Can you work these out from the model? Positions are in its coordinate system, mm. Face numbers are marked on the shaded views. A direction names the side the tool comes from. Coordinates: 2 decimals unless noted, no trailing zeros. Order: outer loops, then holes, each group sorted by start corner. A loop starts at its lowest first (then second) coordinate and runs counter-clockwise, first axis right, second up. Notation, with made-up numbers: (-0.5, 77) -> (34.5, 77) arc R17 cw to (34.5, 87) -> close; hole circle Ø6 at (-22.75, -5). An arc over 180 degrees is marked (long way). Write item = value, one per line.
```python
from build123d import *

# Parameters (mm, degrees)
SKETCH1_W                        = 100
SKETCH1_H                        = 130
BASE_FLANGE1_DEPTH               = 0.7366
BOX_REAR_STRIP_W                 = 4.4196
BOX_REAR_STRIP_H                 = 0.7366
BOX_REAR_STRIP_CUT_DEPTH         = 100
BOX_REAR_DEPTH                   = 100
BOX_FRONT_STRIP_W                = 4.4196
BOX_FRONT_STRIP_H                = 0.7366
BOX_FRONT_STRIP_CUT_DEPTH        = 100
BOX_FRONT_DEPTH                  = 100
BOX_FRONT_TABS_STRIP_W           = 4.4196
BOX_FRONT_TABS_STRIP_H           = 0.7366
BOX_FRONT_TABS_STRIP_CUT_DEPTH   = 59.2634
BOX_FRONT_TABS_STRIP_2_W         = 4.4196
BOX_FRONT_TABS_STRIP_2_H         = 0.7366
BOX_FRONT_TABS_STRIP_CUT_2_DEPTH = 59.2634
BOX_FRONT_TABS_DEPTH             = 59.2634
BOX_FRONT_TABS_BEND_DEPTH        = 59.2634
BOX_REAR_TABS_STRIP_W            = 4.4196
BOX_REAR_TABS_STRIP_H            = 0.7366
BOX_REAR_TABS_STRIP_CUT_DEPTH    = 59.2634
BOX_REAR_TABS_STRIP_2_W          = 4.4196
BOX_REAR_TABS_STRIP_2_H          = 0.7366
BOX_REAR_TABS_STRIP_CUT_2_DEPTH  = 59.2634
BOX_REAR_TABS_DEPTH              = 59.2634
BOX_REAR_TABS_BEND_DEPTH         = 59.2634
EDGE_FLANGE6_DEPTH               = 128.5268
EDGE_FLANGE6_START               = 0.7366
EDGE_FLANGE6_FLAT_DEPTH          = 0.7366
EDGE_FLANGE6_BEND_DEPTH          = 128.5268
EDGE_FLANGE6_FLAT_2_DEPTH        = 0.7366


# Sheet-metal steps are written as plain solids
with BuildPart() as part:
    # Sketch1 → Base-Flange1 (new body)
    with BuildSketch(Plane(origin=(0, 0, 0), x_dir=(1, 0, 0), z_dir=(0, 1, 0))):
        Rectangle(SKETCH1_W, SKETCH1_H)
    extrude(amount=-BASE_FLANGE1_DEPTH)

    # Box rear strip (across the edge) → Box rear strip cut (cut)
    with BuildSketch(Plane(origin=(50, 0, -65), x_dir=(0, 0, 1), z_dir=(-1, 0, 0))):
        with Locations((-1.4732, -0.3683)):
            Rectangle(BOX_REAR_STRIP_W, BOX_REAR_STRIP_H)
    extrude(amount=BOX_REAR_STRIP_CUT_DEPTH, mode=Mode.SUBTRACT)

    # Box rear section (across the edge) → Box rear (add)
    with BuildSketch(Plane(origin=(50, 0, -65), x_dir=(0, 0, 1), z_dir=(-1, 0, 0))):
        with BuildLine():
            Line((-0.7366, 0.7366), (-0.7366, 60))
            Line((-0.7366, 60), (0, 60))
            Line((0, 60), (0, 0.7366))
            ThreePointArc((0, 0.7366), (0.215745145, 0.215745145), (0.7366, 0))
            Line((0.7366, 0), (0.7366, -0.7366))
            ThreePointArc((0.7366, -0.7366), (-0.30510971, -0.30510971), (-0.7366, 0.7366))
        make_face()
    extrude(amount=BOX_REAR_DEPTH)

    # Box front strip (across the edge) → Box front strip cut (cut)
    with BuildSketch(Plane(origin=(-50, 0, 65), x_dir=(0, 0, -1), z_dir=(1, 0, 0))):
        with Locations((-1.4732, -0.3683)):
            Rectangle(BOX_FRONT_STRIP_W, BOX_FRONT_STRIP_H)
    extrude(amount=BOX_FRONT_STRIP_CUT_DEPTH, mode=Mode.SUBTRACT)

    # Box front section (across the edge) → Box front (add)
    with BuildSketch(Plane(origin=(-50, 0, 65), x_dir=(0, 0, -1), z_dir=(1, 0, 0))):
        with BuildLine():
            Line((-0.7366, 0.7366), (-0.7366, 60))
            Line((-0.7366, 60), (0, 60))
            Line((0, 60), (0, 0.7366))
            ThreePointArc((0, 0.7366), (0.215745145, 0.215745145), (0.7366, 0))
            Line((0.7366, 0), (0.7366, -0.7366))
            ThreePointArc((0.7366, -0.7366), (-0.30510971, -0.30510971), (-0.7366, 0.7366))
        make_face()
    extrude(amount=BOX_FRONT_DEPTH)

    # Box-front tabs strip (across the edge) → Box-front tabs strip cut (cut)
    with BuildSketch(Plane(origin=(-50, 0.7366, 65), x_dir=(1, 0, 0), z_dir=(0, 1, 0))):
        with Locations((-1.4732, -0.3683)):
            Rectangle(BOX_FRONT_TABS_STRIP_W, BOX_FRONT_TABS_STRIP_H)
    extrude(amount=BOX_FRONT_TABS_STRIP_CUT_DEPTH, mode=Mode.SUBTRACT)

    # Box-front tabs strip 2 (across the edge) → Box-front tabs strip cut 2 (cut)
    with BuildSketch(Plane(origin=(50, 60, 65), x_dir=(-1, 0, 0), z_dir=(0, -1, 0))):
        with Locations((-1.4732, -0.3683)):
            Rectangle(BOX_FRONT_TABS_STRIP_2_W, BOX_FRONT_TABS_STRIP_2_H)
    extrude(amount=BOX_FRONT_TABS_STRIP_CUT_2_DEPTH, mode=Mode.SUBTRACT)

    # Box-front tabs section (across the edge) → Box-front tabs (add)
    with BuildSketch(Plane(origin=(-50, 0.7366, 65), x_dir=(1, 0, 0), z_dir=(0, 1, 0))):
        with BuildLine():
            Line((-0.7366, 0.7366), (-0.7366, 10))
            Line((-0.7366, 10), (0, 10))
            Line((0, 10), (0, 0.7366))
            ThreePointArc((0, 0.7366), (0.215745145, 0.215745145), (0.7366, 0))
            Line((0.7366, 0), (0.7366, -0.7366))
            ThreePointArc((0.7366, -0.7366), (-0.30510971, -0.30510971), (-0.7366, 0.7366))
        make_face()
    extrude(amount=BOX_FRONT_TABS_DEPTH)

    # Box-front tabs section 2 (across the edge) → Box-front tabs bend (add)
    with BuildSketch(Plane(origin=(50, 60, 65), x_dir=(-1, 0, 0), z_dir=(0, -1, 0))):
        with BuildLine():
            Line((-0.7366, 0.7366), (-0.7366, 10))
            Line((-0.7366, 10), (0, 10))
            Line((0, 10), (0, 0.7366))
            ThreePointArc((0, 0.7366), (0.215745145, 0.215745145), (0.7366, 0))
            Line((0.7366, 0), (0.7366, -0.7366))
            ThreePointArc((0.7366, -0.7366), (-0.30510971, -0.30510971), (-0.7366, 0.7366))
        make_face()
    extrude(amount=BOX_FRONT_TABS_BEND_DEPTH)

    # Box-rear tabs strip (across the edge) → Box-rear tabs strip cut (cut)
    with BuildSketch(Plane(origin=(50, 0.7366, -65), x_dir=(-1, 0, 0), z_dir=(0, 1, 0))):
        with Locations((-1.4732, -0.3683)):
            Rectangle(BOX_REAR_TABS_STRIP_W, BOX_REAR_TABS_STRIP_H)
    extrude(amount=BOX_REAR_TABS_STRIP_CUT_DEPTH, mode=Mode.SUBTRACT)

    # Box-rear tabs strip 2 (across the edge) → Box-rear tabs strip cut 2 (cut)
    with BuildSketch(Plane(origin=(-50, 60, -65), x_dir=(1, 0, 0), z_dir=(0, -1, 0))):
        with Locations((-1.4732, -0.3683)):
            Rectangle(BOX_REAR_TABS_STRIP_2_W, BOX_REAR_TABS_STRIP_2_H)
    extrude(amount=BOX_REAR_TABS_STRIP_CUT_2_DEPTH, mode=Mode.SUBTRACT)

    # Box-rear tabs section (across the edge) → Box-rear tabs (add)
    with BuildSketch(Plane(origin=(50, 0.7366, -65), x_dir=(-1, 0, 0), z_dir=(0, 1, 0))):
        with BuildLine():
            Line((-0.7366, 0.7366), (-0.7366, 10))
            Line((-0.7366, 10), (0, 10))
            Line((0, 10), (0, 0.7366))
            ThreePointArc((0, 0.7366), (0.215745145, 0.215745145), (0.7366, 0))
            Line((0.7366, 0), (0.7366, -0.7366))
            ThreePointArc((0.7366, -0.7366), (-0.30510971, -0.30510971), (-0.7366, 0.7366))
        make_face()
    extrude(amount=BOX_REAR_TABS_DEPTH)

    # Box-rear tabs section 2 (across the edge) → Box-rear tabs bend (add)
    with BuildSketch(Plane(origin=(-50, 60, -65), x_dir=(1, 0, 0), z_dir=(0, -1, 0))):
        with BuildLine():
            Line((-0.7366, 0.7366), (-0.7366, 10))
            Line((-0.7366, 10), (0, 10))
            Line((0, 10), (0, 0.7366))
            ThreePointArc((0, 0.7366), (0.215745145, 0.215745145), (0.7366, 0))
            Line((0.7366, 0), (0.7366, -0.7366))
            ThreePointArc((0.7366, -0.7366), (-0.30510971, -0.30510971), (-0.7366, 0.7366))
        make_face()
    extrude(amount=BOX_REAR_TABS_BEND_DEPTH)

    # Edge-Flange6 bend section (across the edge) → Edge-Flange6 (add)
    with BuildSketch(Plane(origin=(-51.2366, 0, -64.2634), x_dir=(1, 0, 0), z_dir=(0, 0, 1))):
        with BuildLine():
            Line((-0.7366, 0.7366), (0, 0.7366))
            ThreePointArc((0, 0.7366), (0.215745145, 0.215745145), (0.7366, 0))
            Line((0.7366, 0), (1.2366, 0))
            Line((1.2366, 0), (1.2366, -0.7366))
            Line((1.2366, -0.7366), (0.7366, -0.7366))
            ThreePointArc((0.7366, -0.7366), (-0.30510971, -0.30510971), (-0.7366, 0.7366))
        make_face()
    extrude(amount=EDGE_FLANGE6_DEPTH)

    # Edge-Flange6 profile (on flange) → Edge-Flange6 flat (add)
    with BuildSketch(Plane.ZY.offset(51.2366).offset(EDGE_FLANGE6_START)):
        Polygon((-64.2634, 60), (-64.2634, 0.7366), (64.2634, 0.7366), (64.2634, 60), (2.12, 60), (2.12, 55), (-2.12, 55), (-2.12, 60), align=None)
    extrude(amount=-EDGE_FLANGE6_FLAT_DEPTH)

    # Edge-Flange6 bend section 2 (across the edge) → Edge-Flange6 bend (add)
    with BuildSketch(Plane(origin=(51.2366, 0, 64.2634), x_dir=(-1, 0, 0), z_dir=(0, 0, -1))):
        with BuildLine():
            Line((-0.7366, 0.7366), (0, 0.7366))
            ThreePointArc((0, 0.7366), (0.215745145, 0.215745145), (0.7366, 0))
            Line((0.7366, 0), (1.2366, 0))
            Line((1.2366, 0), (1.2366, -0.7366))
            Line((1.2366, -0.7366), (0.7366, -0.7366))
            ThreePointArc((0.7366, -0.7366), (-0.30510971, -0.30510971), (-0.7366, 0.7366))
        make_face()
    extrude(amount=EDGE_FLANGE6_BEND_DEPTH)

    # Edge-Flange6 profile 2 (on flange) → Edge-Flange6 flat 2 (add)
    with BuildSketch(Plane(origin=(51.2366, 0, 0), x_dir=(0, 0, -1), z_dir=(1, 0, 0)).offset(EDGE_FLANGE6_START)):
        Polygon((-64.2634, 60), (-64.2634, 0.7366), (64.2634, 0.7366), (64.2634, 60), (2.12, 60), (2.12, 55), (-2.12, 55), (-2.12, 60), align=None)
    extrude(amount=-EDGE_FLANGE6_FLAT_2_DEPTH)


solid = part.part
```
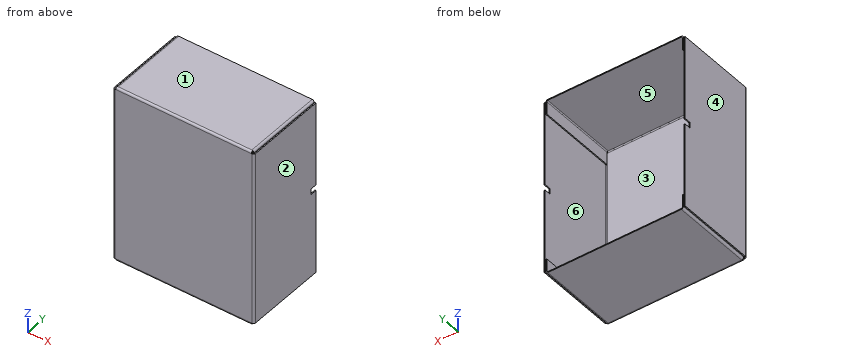
Item 1: I want a section at A-A, the plane y = 45. Give the number of separate pieces and of enclosed holes in the cut face, plus the area to 3 significant figures.
A:
separate_pieces = 4
enclosed_holes = 0
area = 367 mm2
Item 2: If I drill on probe 1 along X at (y, z) = (48, 56); probe 2 along X at (y, z) = (10.5, 14); probe 3 along Z at (x, y) = (-12.5, 31), over which ranges is the centre line in solid material (lowest first)?
A:
probe_1 = -51.97 to -51.24, -50.74 to -50, 50 to 50.74, 51.24 to 51.97
probe_2 = -51.97 to -51.24, 51.24 to 51.97
probe_3 = -65.74 to -65, 65 to 65.74
Item 3: I want a section at B-B, the plane z = 40.5. Please give me the cut outline in (x, y), plus the area to 3 significant figures.
A:
outline = (-51.97, 0.74) arc R1.47 ccw to (-50.5, -0.74) -> (50.5, -0.74) arc R1.47 ccw to (51.97, 0.74) -> (51.97, 60) -> (51.24, 60) -> (51.24, 0.74) arc R0.74 cw to (50.5, 0) -> (-50.5, 0) arc R0.74 cw to (-51.24, 0.74) -> (-51.24, 60) -> (-51.97, 60) -> close
area = 164 mm2
Item 4: I want a section at C-C, the plane x = -6.5. Please give me the cut outline in (y, z).
A:
outline = (-0.74, -64.26) arc R1.47 ccw to (0.74, -65.74) -> (60, -65.74) -> (60, -65) -> (0.74, -65) arc R0.74 cw to (0, -64.26) -> (0, 64.26) arc R0.74 cw to (0.74, 65) -> (60, 65) -> (60, 65.74) -> (0.74, 65.74) arc R1.47 ccw to (-0.74, 64.26) -> close
Item 5: For the marked faces 4, 5 and 6, which set-ups out of +Z, -Z, +X, -X, +Y, -Y let a thin tool reach every point of the face, with its end or its side?
A:
face_4 = +Z, -Z, -X, +Y, -Y
face_5 = +Y
face_6 = +Z, -Z, +Y
Item 6: I'm going to push flat-ended pins straight in: P1, Ø2, axis at x = 20.5, z = 20.5, coming from the +Y side; P2, Ø0.6, axis at x = 51.5, y = 44, coming from the +Z side; P3, Ø1.2, axis at y = 0, z = -65, coming from the +X side. Where does each tip first touch, or does it pass through?
A:
P1 = 0
P2 = 64.26
P3 = 50
Item 7: If we mould it in two halves opening along X, with no side actions, what happens to the marked faces 1, 2 and 3? For each: pulls with the +X half, pulls with the -X half, needs draft (parallel to the pull), parting line crosses it, or undercut.
A:
face_1 = needs draft
face_2 = pulls with the +X half
face_3 = undercut
